Read the model definition and answer for the solid it produces. Units are mm, in the model's axes. A direction names the side the tool comes from. Coordinates: 2 decimals unless noted, no trailing zeros. Write each loop counter-clockwise with the first axis right and the second up, starting at its lowest first coordinate (ties: lowest second). Pieces come first, ordered by that corner, then holes.
from build123d import *

# Parameters (mm, degrees)
BOSS_EXTRUDE1_START = 76.2
SKETCH2_R           = 152.4
SKETCH2_R_2         = 50.8
BOSS_EXTRUDE1_DEPTH = 25.4
BOSS_EXTRUDE2_START = 203.2
SKETCH3_R           = 152.4
SKETCH3_R_2         = 139.7
BOSS_EXTRUDE2_DEPTH = 203.2
BOSS_EXTRUDE3_START = 6.35
SKETCH4_R           = 152.4
BOSS_EXTRUDE3_DEPTH = 6.35
CUT_EXTRUDE1_START  = -120.65
CUT_EXTRUDE1_DEPTH  = 6.35


with BuildPart() as part:
    # Sketch2 → Boss-Extrude1 (new body)
    with BuildSketch(Plane(origin=(0, 0, 0), x_dir=(0, 0, -1), z_dir=(1, 0, 0)).offset(BOSS_EXTRUDE1_START)):
        Circle(SKETCH2_R)
        Circle(SKETCH2_R_2, mode=Mode.SUBTRACT)
    extrude(amount=BOSS_EXTRUDE1_DEPTH)

    # Sketch3 → Boss-Extrude2 (add)
    with BuildSketch(Plane.ZY.offset(-76.2).offset(BOSS_EXTRUDE2_START)):
        Circle(SKETCH3_R)
        Circle(SKETCH3_R_2, mode=Mode.SUBTRACT)
    extrude(amount=-BOSS_EXTRUDE2_DEPTH)

    # Sketch4 → Boss-Extrude3 (add)
    with BuildSketch(Plane.ZY.offset(127).offset(BOSS_EXTRUDE3_START)):
        Circle(SKETCH4_R)
    extrude(amount=-BOSS_EXTRUDE3_DEPTH)

    # Sketch5 → Cut-Extrude1 (cut)
    with BuildSketch(Plane.ZY.offset(254).offset(CUT_EXTRUDE1_START)):
        with BuildLine():
            Line((19.05, 88.9), (19.05, -88.9))
            ThreePointArc((19.05, -88.9), (-6.35, -114.3), (-31.75, -88.9))
            Line((-31.75, -88.9), (-31.75, 88.9))
            ThreePointArc((-31.75, 88.9), (-6.35, 114.3), (19.05, 88.9))
        make_face()
    extrude(amount=-CUT_EXTRUDE1_DEPTH, mode=Mode.SUBTRACT)


solid = part.part
Item 1: Given pin 1 (10 mm diameter, centred on x = -67, y = -82, fed in from -Z); pin 2 (1.5 mm diameter, centred on x = 53.5, z = 105.5, fed in from -Y); pin 3 (6 mm diameter, centred on x = -78.5, y = 31.5, fed in from -Z), each flat-ended and moving along its own axis, determine where each tip first touches the part or whether it passes through.
Item 2: The part is cut by section B-B (y = -13.5). Give the vertices of the cut face in (x, z).
Item 3: Determine the mould class of faces 5 (the cylindrical face through (-26.82, -85.01, -110.86)), 6 (the flat face through (101.6, 2, -66)) for opening direction Z: +Z half, -Z half, draft (parallel to the pull), parting line (faces both ways), or undercut.
Item 4: The part is cut by section D-D (x = 46). Give the vertices of the cut face in (y, z).
Item 5: For faces 1 (the cylindrical face through (88.722, -49.592, 11.012)), 2 (the cylindrical face through (-130.219, 114.294, -6.909)), 3 (the flat face through (-127, 2, 29)), 4 (the flat face through (-133.35, 2, 32)), determine the directions among +Z, -Z, +X, -X, +Y, -Y from which every point of the face is accessible in a straight line to the end or side of a thin tool.
Item 6: The part is cut by section A-A (z = 59.5). Give the vertices of the cut face in (x, y), and give its area (3 significant figures).
Item 7: The part is cut by section C-C (z = -6.35). Give the vertices of the cut face in (x, y), and give its area (3 significant figures).
Item 8: Find the intervals of material crossed by probe 1 along X at (y, z) = (17, -118); probe 2 along Y at (x, z) = (86.75, 0); probe 3 along Y at (x, z) = (-80, 0), in increasing order.
Answer:
1. pin 1: stops at z = -131.52
1. pin 2: stops at y = -110.69
1. pin 3: stops at z = -149.71
2. outline: (-133.35, -151.8) - (101.6, -151.8) - (101.6, -48.97) - (76.2, -48.97) - (76.2, -139.05) - (-127, -139.05) - (-127, -31.75) - (-133.35, -31.75) - close; (-133.35, 19.05) - (-127, 19.05) - (-127, 139.05) - (76.2, 139.05) - (76.2, 48.97) - (101.6, 48.97) - (101.6, 151.8) - (-133.35, 151.8) - close
3. face 5: undercut
3. face 6: draft
4. outline: circle Ø304.8 at (0, 0); hole circle Ø279.4 at (0, 0)
5. face 1: +X
5. face 2: -X
5. face 3: none
5. face 4: +Z, -Z, -X, +Y, -Y
6. outline: (-133.35, -140.31) - (101.6, -140.31) - (101.6, 140.31) - (-133.35, 140.31) - close; hole (-127, -126.4) - (76.2, -126.4) - (76.2, 126.4) - (-127, 126.4) - close
6. area: 14,600 mm2
7. outline: (-133.35, -152.27) - (101.6, -152.27) - (101.6, -50.4) - (76.2, -50.4) - (76.2, -139.56) - (-127, -139.56) - (-127, -114.3) - (-133.35, -114.3) - close; (-133.35, 114.3) - (-127, 114.3) - (-127, 139.56) - (76.2, 139.56) - (76.2, 50.4) - (101.6, 50.4) - (101.6, 152.27) - (-133.35, 152.27) - close
7. area: 10,800 mm2
8. probe 1: x = -133.35 to -127, 76.2 to 101.6
8. probe 2: y = -152.4 to -50.8, 50.8 to 152.4
8. probe 3: y = -152.4 to -139.7, 139.7 to 152.4
